Geometry: final body of the model. Coordinates: model frame, mm. Face numbers are marked on the shaded views. A direction names the side the tool comes from. Coordinates: 2 decimals unless noted, no trailing zeros. Write each loop counter-clockwise with the first axis right and the second up, starting at its lowest first coordinate (ties: lowest second). Pieces come first, ordered by that corner, then holes. Notation, with made-up numbers: (37.5, -38) -> (56.5, -38) arc R13 ccw to (56.5, -22) -> close; hole circle Ø5 at (-37.5, 35.5). An arc over 180 degrees is marked (long way). Answer as a JSON object with one key per item and string values. Group by question number.
```python
from build123d import *

# Parameters (mm, degrees)
SKETCH1_W           = 50.8
SKETCH1_H           = 25.4
SKETCH1_W_2         = 45.72
SKETCH1_H_2         = 20.32
BOSS_EXTRUDE1_DEPTH = 25.4
SKETCH3_R           = 3.048
CUT_EXTRUDE1_DEPTH  = 63.217039467
SKETCH4_R           = 2.54
CUT_EXTRUDE2_DEPTH  = 63.217039467


with BuildPart() as part:
    # Sketch1 → Boss-Extrude1 (new body)
    with BuildSketch(Plane(origin=(0, 0, 0), x_dir=(0, 0, -1), z_dir=(1, 0, 0))):
        with Locations((25.4, 12.7)):
            Rectangle(SKETCH1_W, SKETCH1_H)
        with Locations((25.4, 12.7)):
            Rectangle(SKETCH1_W_2, SKETCH1_H_2, mode=Mode.SUBTRACT)
    extrude(amount=BOSS_EXTRUDE1_DEPTH)

    # Sketch3 → Cut-Extrude1 (cut, through all)
    with BuildSketch(Plane(origin=(0, 25.4, 0), x_dir=(1, 0, 0), z_dir=(0, 1, 0))):
        with Locations(Location((12.7, 34.798, 0), (0, 0, 270))):
            Circle(SKETCH3_R)
    extrude(amount=-CUT_EXTRUDE1_DEPTH, mode=Mode.SUBTRACT)

    # Sketch4 → Cut-Extrude2 (cut, through all)
    with BuildSketch(Plane.XY):
        with Locations((12.7, 12.7)):
            Circle(SKETCH4_R)
    extrude(amount=-CUT_EXTRUDE2_DEPTH, mode=Mode.SUBTRACT)


solid = part.part
```
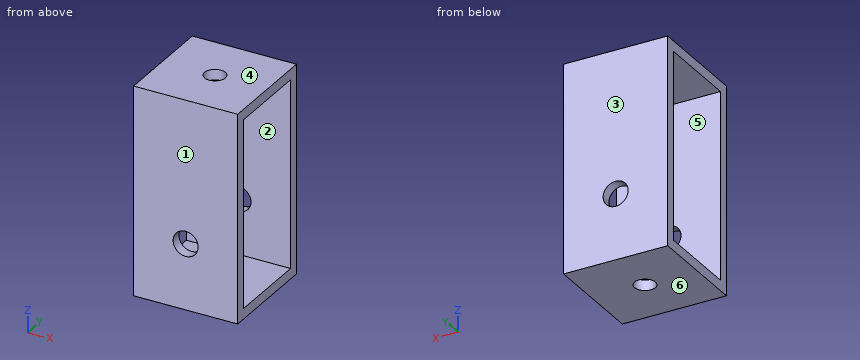
Item 1: Ray query, L1, parallel to Y at x = 13.5, z = -48; L2, parallel to Y at x = 12.7, z = -49.4; L3, parallel to Z at x = 7, y = 22.5. Return the intervals inside material, ascending. Write a range as [from, to].
Item 2: Section A-A on x = 12.7. Output: boundary loops of the cut face in (y, z), then the cut area to 3 significant figures.
Item 3: Mould query, pull axis Z, two halves, no side actions, for the marked faces 3, 4, 5 and 6. Classes: +Z half, -Z half, draft (parallel to the pull), parting line (faces both ways), or undercut.
Item 4: Section C-C on y = 6.75. Output: boundary loops of the cut face in (x, z).
Item 5: Set-up query: the marked faces 1 and 2. Return all of +Z, -Z, +X, -X, +Y, -Y with unobstructed straight access to the full face (end or side cutting, diameter ignored); none if empty.
Item 6: Section B-B on y = 12.7. Output: boundary loops of the cut face in (x, z), then the cut area to 3 significant figures.
Item 7: Contact query for a flat-ended pin moving along its axis: pin 1 (3.5 mm diameter, centred on x = 12.7, z = -34.798, fed in from -Y). Output: stop coordinate, or through.
Item 8: Section D-D on z = -40. Output: boundary loops of the cut face in (x, y).
Answer sheet:
{
 "1": {"L1": "y = [0, 2.54], [22.86, 25.4]", "L2": "y = [0, 10.16], [15.24, 25.4]", "L3": "z = [-50.8, -48.26], [-2.54, 0]"},
 "2": {"outline": "(0, -50.8) -> (10.16, -50.8) -> (10.16, -48.26) -> (2.54, -48.26) -> (2.54, -37.85) -> (0, -37.85) -> close; (0, -31.75) -> (2.54, -31.75) -> (2.54, -2.54) -> (10.16, -2.54) -> (10.16, 0) -> (0, 0) -> close; (15.24, -50.8) -> (25.4, -50.8) -> (25.4, -37.85) -> (22.86, -37.85) -> (22.86, -48.26) -> (15.24, -48.26) -> close; (15.24, -2.54) -> (22.86, -2.54) -> (22.86, -31.75) -> (25.4, -31.75) -> (25.4, 0) -> (15.24, 0) -> close", "area": "305 mm^2"},
 "3": {"face 3": "draft", "face 4": "+Z half", "face 5": "undercut", "face 6": "-Z half"},
 "4": {"outline": "(0, -50.8) -> (25.4, -50.8) -> (25.4, -48.26) -> (0, -48.26) -> close; (0, -2.54) -> (25.4, -2.54) -> (25.4, 0) -> (0, 0) -> close"},
 "5": {"face 1": "+Z, -Z, +X, -X, -Y", "face 2": "+X, -X"},
 "6": {"outline": "(0, -50.8) -> (10.16, -50.8) -> (10.16, -48.26) -> (0, -48.26) -> close; (0, -2.54) -> (10.16, -2.54) -> (10.16, 0) -> (0, 0) -> close; (15.24, -50.8) -> (25.4, -50.8) -> (25.4, -48.26) -> (15.24, -48.26) -> close; (15.24, -2.54) -> (25.4, -2.54) -> (25.4, 0) -> (15.24, 0) -> close", "area": "103 mm^2"},
 "7": {"pin 1": "passes through"},
 "8": {"outline": "(0, 0) -> (25.4, 0) -> (25.4, 2.54) -> (0, 2.54) -> close; (0, 22.86) -> (25.4, 22.86) -> (25.4, 25.4) -> (0, 25.4) -> close"}
}
